Input: part model. Units: mm. Frame: model coordinates. A direction names the side the tool comes from. Give positions to 0.01 mm unless a question says otherwise; leave off trailing zeros. Order: outer loops, then holes, each group sorted by start corner. A loop starts at its lowest first (then second) coordinate and runs counter-clockwise, first axis right, second up.
```python
from build123d import *

# Parameters (mm, degrees)
BOSS_EXTRUDE1_DEPTH = 25
CUT_EXTRUDE1_DEPTH  = 10
SKETCH6_R           = 11
CUT_EXTRUDE2_DEPTH  = 10
BOSS_EXTRUDE2_DEPTH = 2.5


with BuildPart() as part:
    # Sketch1 → Boss-Extrude1 (new body, symmetric)
    with BuildSketch(Plane.XY):
        Polygon((53, 0), (0, 0), (0, 51), (2.5, 51), (2.5, 2.5), (53, 2.5), align=None)
    extrude(amount=BOSS_EXTRUDE1_DEPTH, both=True)

    # Sketch5 → Cut-Extrude1 (cut)
    with BuildSketch(Plane(origin=(0, 2.5, 0), x_dir=(1, 0, 0), z_dir=(0, 1, 0))):
        with BuildLine():
            Line((13.25, 17), (41.75, 17))
            ThreePointArc((41.75, 17), (44, 14.75), (41.75, 12.5))
            Line((41.75, 12.5), (13.25, 12.5))
            ThreePointArc((13.25, 12.5), (11, 14.75), (13.25, 17))
        make_face()
        with BuildLine():
            Line((13.25, -12.5), (41.75, -12.5))
            ThreePointArc((41.75, -12.5), (44, -14.75), (41.75, -17))
            Line((41.75, -17), (13.25, -17))
            ThreePointArc((13.25, -17), (11, -14.75), (13.25, -12.5))
        make_face()
    extrude(amount=-CUT_EXTRUDE1_DEPTH, mode=Mode.SUBTRACT)

    # Sketch6 → Cut-Extrude2 (cut)
    with BuildSketch(Plane(origin=(2.5, 0, 0), x_dir=(0, 0, -1), z_dir=(1, 0, 0))):
        with Locations((0, 30)):
            Circle(SKETCH6_R)
    extrude(amount=-CUT_EXTRUDE2_DEPTH, mode=Mode.SUBTRACT)

    # Sketch7 → Boss-Extrude2 (add)
    with BuildSketch(Plane.XY.offset(25)):
        Polygon((2.5, 22), (16, 2.5), (2.5, 2.5), align=None)
    boss_extrude2 = extrude(amount=-BOSS_EXTRUDE2_DEPTH)

    # Mirror1: Boss-Extrude2 across plane
    add(boss_extrude2.mirror(Plane.XY))


solid = part.part
```
1) First-contact query: P1, Ø1, axis at y = 23, z = 16, coming from the +X side; P2, Ø6, axis at x = 38, z = -2, coming from the -Y side; P3, Ø8, axis at y = 32, z = -3.5, coming from the +X side; P4, Ø8, axis at x = 13.5, z = 7, coming from the +Y side. Flat tips, straight axial feed; report the tip coordinate or a pass-through.
2) Line query: probe 1 along Z at (x, y) = (6, 8.5); probe 2 along Y at (x, z) = (1, 0); probe 3 along X at (y, z) = (48, 20.5). Output: solid intervals per line, ascending.
3) Cut plane A-A (z = 0). Return the cut outline in (x, y), then the cut area to 3 significant figures.
4) Cut plane B-B (x = 39). Return the cut outline in (y, z).
5) Cut plane C-C (y = 21). Return the cut outline in (x, z), then the cut area to 3 significant figures.
6) Pull-direction query (Z, two-part tool) for faces 4 (the face through (9, 11, 25)), 5 (the face through (11, 1.3, -14.7)), 6 (the face through (53, 1, 0)), 7 (the face through (27, 1, 12.5)); classes: pulls with the +Z half, pulls with the -Z half, needs draft (parallel to the pull), parting line crosses it, or undercut.
7) Cut plane D-D (x = 8.5). Return the cut outline in (y, z).
8) Reachability of faces 1 (the face through (27, 1, -17)), 2 (the face through (1, 51, 0)), 3 (the face through (2.5, 27, -11)) from +Z, -Z, +X, -X, +Y, -Y: full face, straight path, thin tool, end or side. Return the list, or none.
Geometry says:
1. P1: stops at x = 2.5
1. P2: stops at y = 0
1. P3: passes through
1. P4: stops at y = 2.5
2. probe 1: z = -25 to -22.5, 22.5 to 25
2. probe 2: y = 0 to 19, 41 to 51
2. probe 3: x = 0 to 2.5
3. outline: (0, 0) - (53, 0) - (53, 2.5) - (2.5, 2.5) - (2.5, 19) - (0, 19) - close; (0, 41) - (2.5, 41) - (2.5, 51) - (0, 51) - close
3. area: 199 mm2
4. outline: (0, -25) - (2.5, -25) - (2.5, -17) - (0, -17) - close; (0, -12.5) - (2.5, -12.5) - (2.5, 12.5) - (0, 12.5) - close; (0, 17) - (2.5, 17) - (2.5, 25) - (0, 25) - close
5. outline: (0, -25) - (3.19, -25) - (3.19, -22.5) - (2.5, -22.5) - (2.5, -6.32) - (0, -6.32) - close; (0, 6.32) - (2.5, 6.32) - (2.5, 22.5) - (3.19, 22.5) - (3.19, 25) - (0, 25) - close
5. area: 96.8 mm2
6. face 4: pulls with the +Z half
6. face 5: undercut
6. face 6: needs draft
6. face 7: undercut
7. outline: (0, -25) - (13.33, -25) - (13.33, -22.5) - (2.5, -22.5) - (2.5, 22.5) - (13.33, 22.5) - (13.33, 25) - (0, 25) - close
8. face 1: +Y, -Y
8. face 2: +Z, -Z, +X, -X, +Y
8. face 3: +X, +Y
